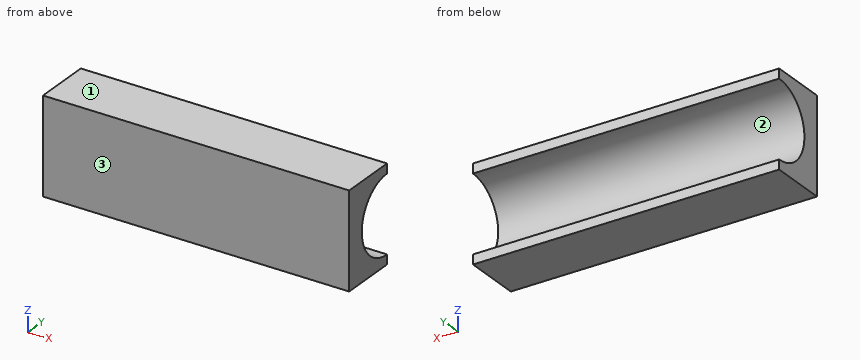
Autodesk Inventor part; units mm, degrees
ref_plane "YZ Plane" through (0, 0, 0) normal (1, 0, 0) x (0, 1, 0)
ref_plane "XZ Plane" through (0, 0, 0) normal (0, 1, 0) x (-1, 0, 0)
ref_plane "XY Plane" through (0, 0, 0) normal (0, 0, 1) x (1, 0, 0)
sketch "Sketch1" plane through (0, 0, 0) normal (1, 0, 0) x (0, 1, 0)
  line L0 (19.05, -2.1167) -> (0, -2.1167)
  line L1 (0, -2.1167) -> (0, -33.8667)
  line L2 (0, -33.8667) -> (19.05, -33.8667)
  arc A0 (19.05, -5.2917) -> (19.05, -30.6917) centre (19.05, -17.9917) ccw
  line L3 (19.05, -33.8667) -> (19.05, -30.6917)
  line L4 (19.05, -5.2917) -> (19.05, -2.1167)
  point P0 (0, 0)
  dimension "d0" = 12.7
  dimension "d1" = 19.05
  dimension "d2" = 31.75
  dimension "d3" = 19.05
  dimension "d4" = 19.05
extrude "Extrusion1" add sketch "Sketch1" along normal blind 101.6
properties part number "Ball Ramp - Goldberg"
Verification items for the finished model (mm, model axes). Face numbers are marked on the shaded views. Coordinates: 2 decimals unless noted, no trailing zeros. Write each loop counter-clockwise with the first axis right and the second up, starting at its lowest first coordinate (ties: lowest second). Pieces come first, ordered by that corner, then holes. Notation, with made-up numbers: (-11, 24) - (3, 24) arc R11 ccw to (3, 33) - close; hole circle Ø11 at (-8.75, 72). An arc over 180 degrees is marked (long way). Answer as a JSON object with one key per item and string values.
(1) Cross-section at D-D on z = -15.5. Record the cut outline in (x, y).
Report:
{"outline": "(0, 0) - (101.6, 0) - (101.6, 6.6) - (0, 6.6) - close"}
(2) Mould release check, pull along Z, two halves, no side actions. Record for the marked faces 1, 2 and 3: pulls with the +Z half, pulls with the -Z half, needs draft (parallel to the pull), parting line crosses it, or undercut.
Report:
{"face 1": "pulls with the +Z half", "face 2": "undercut", "face 3": "needs draft"}
(3) Cross-section at A-A on y = 17.5. Record the cut outline in (x, z), plus the area to 3 significant figures.
Report:
{"outline": "(0, -33.87) - (101.6, -33.87) - (101.6, -30.6) - (0, -30.6) - close; (0, -5.39) - (101.6, -5.39) - (101.6, -2.12) - (0, -2.12) - close", "area": "664 mm^2"}
(4) Thickness scan on line 1 along Z through (x, y) = (91.5, 11.5); line 2 along Z through (x, y) = (52, 9.25); line 3 along Y through (x, z) = (73, -17.5). Record the ranges inside material, lowest first.
Report:
{"line 1": "-33.87 to -28.2, -7.78 to -2.12", "line 2": "-33.87 to -26.07, -9.91 to -2.12", "line 3": "0 to 6.36"}
(5) Cross-section at B-B on x = 79.5. Record the cut outline in (y, z), plus the area to 3 significant figures.
Report:
{"outline": "(0, -33.87) - (19.05, -33.87) - (19.05, -30.69) arc R12.7 cw to (19.05, -5.29) - (19.05, -2.12) - (0, -2.12) - close", "area": "351 mm^2"}
(6) Cross-section at C-C on y = 8.75. Record the cut outline in (x, z), plus the area to 3 significant figures.
Report:
{"outline": "(0, -33.87) - (101.6, -33.87) - (101.6, -25.42) - (0, -25.42) - close; (0, -10.56) - (101.6, -10.56) - (101.6, -2.12) - (0, -2.12) - close", "area": "1,720 mm^2"}
